Input: part model. Units: mm. Frame: model coordinates. Face numbers are marked on the shaded views. A direction names the side the tool comes from. Coordinates: 2 decimals unless noted, no trailing zeros. Loops run counter-clockwise (first coordinate to the right, second up) from the corner with the lowest first, then second, coordinate; pieces in that order, holes last. Notation, with made-up numbers: M -4,-7.5 L 29,-7.5 A8 ccw 29,7.5 Z; hole C 9,43 d6. An arc over 180 degrees is marked long. Use a Markdown table: item, result. Add a question column.
1. Section C-C on x = 13. Output: boundary loops of the cut face in (y, z), then the cut area to 3 significant figures.
2. Section D-D on y = 11. Output: boundary loops of the cut face in (x, z), then the cut area to 3 significant figures.
3. Section B-B on z = -2.5. Output: boundary loops of the cut face in (x, y).
4. Section A-A on y = 2.25. Output: boundary loops of the cut face in (x, z).
5. Line query: L1, parallel to X at y = 18, z = 8.5; L2, parallel to Y at x = 16, z = -8.5; L3, parallel to X at y = 3.75, z = 6.5. Output: solid intervals per line, ascending. Write a range as [from, to].
6. Set-up query: the marked faces 1, 2 and 3. Return all of +Z, -Z, +X, -X, +Y, -Y with unobstructed straight access to the full face (end or side cutting, diameter ignored); none if empty.
7. Pin query (flat end, axial travel): pin 1 (5.5 mm diameter, centred on x = 19.5, y = 3, fed in from +Z); pin 2 (10 mm diameter, centred on y = 17.5, z = 7.5, fed in from +X); pin 3 (10 mm diameter, centred on y = 10, z = 3.5, fed in from +X). Return the tip coordinate at first contact, or that it passes through.
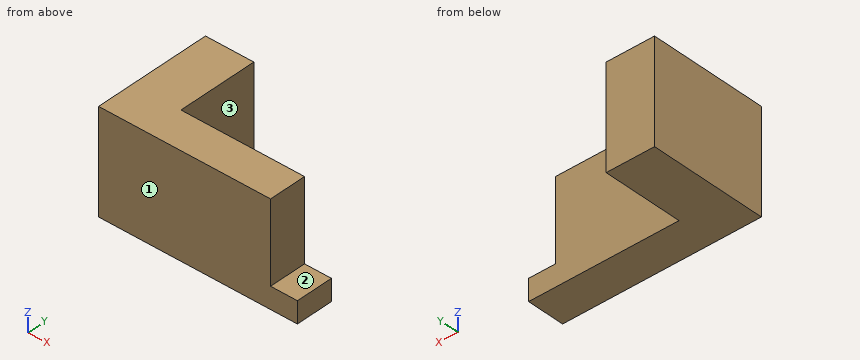
```python
from build123d import *

# Parameters (mm, degrees)
SKETCH1_W           = 32
SKETCH1_H           = 19
BOSS_EXTRUDE1_DEPTH = 7
SKETCH2_W           = 9
SKETCH2_H           = 19
BOSS_EXTRUDE2_DEPTH = 15
SKETCH3_W           = 4
SKETCH3_H           = 7
BOSS_EXTRUDE3_DEPTH = 5


with BuildPart() as part:
    # Sketch1 → Boss-Extrude1 (new body)
    with BuildSketch(Plane(origin=(0, 0, 0), x_dir=(1, 0, 0), z_dir=(0, 1, 0))):
        Rectangle(SKETCH1_W, SKETCH1_H)
    extrude(amount=BOSS_EXTRUDE1_DEPTH)

    # Sketch2 → Boss-Extrude2 (add)
    with BuildSketch(Plane(origin=(0, 7, 0), x_dir=(1, 0, 0), z_dir=(0, 1, 0))):
        with Locations((-11.5, 0)):
            Rectangle(SKETCH2_W, SKETCH2_H)
    extrude(amount=BOSS_EXTRUDE2_DEPTH)

    # Sketch3 → Boss-Extrude3 (add)
    with BuildSketch(Plane(origin=(16, 0, 0), x_dir=(0, 0, -1), z_dir=(1, 0, 0))):
        with Locations((7.5, 3.5)):
            Rectangle(SKETCH3_W, SKETCH3_H)
    extrude(amount=BOSS_EXTRUDE3_DEPTH)


solid = part.part
```
Answers below:
| question | item | result |
|---|---|---|
| 1 | outline | M 0,-9.5 L 7,-9.5 L 7,9.5 L 0,9.5 Z |
| 1 | area | 133 mm² |
| 2 | outline | M -16,-9.5 L -7,-9.5 L -7,9.5 L -16,9.5 Z |
| 2 | area | 171 mm² |
| 3 | outline | M -16,0 L 16,0 L 16,7 L -7,7 L -7,22 L -16,22 Z |
| 4 | outline | M -16,-9.5 L 21,-9.5 L 21,-5.5 L 16,-5.5 L 16,9.5 L -16,9.5 Z |
| 5 | L1 | x = [-16, -7] |
| 5 | L2 | y = [0, 7] |
| 5 | L3 | x = [-16, 16] |
| 6 | face 1 | +Z, -Z, +X, -X, -Y |
| 6 | face 2 | +Z, +X, +Y, -Y |
| 6 | face 3 | +Z, -Z, +X, +Y |
| 7 | pin 1 | stops at z = -5.5 |
| 7 | pin 2 | stops at x = -7 |
| 7 | pin 3 | stops at x = 16 |
